For this review, take the finished solid that the model builds, in its own axes (mm). A direction names the side the tool comes from. Round coordinates to 2 decimals unless told otherwise and drop trailing zeros. Write each loop counter-clockwise with the first axis right and the second up, starting at its lowest first coordinate (ties: lowest second). Pieces come first, ordered by that corner, then holes. Notation, with made-up numbers: (32, -16.5) - (78, -16.5) arc R18 ccw to (78, 4.5) - close; hole circle Ø6 at (70, 50.5). An arc over 180 degrees is marked (long way). Answer in a Markdown table with one row per item. Add a question column.
from build123d import *

# Parameters (mm, degrees)
F0_W      = 54.494548589
F0_H      = 39.0236377716
F1_DEPTH  = 5.08
F3_DEPTH  = 12.7
F4_W      = 28.1709115952
F4_H      = 15.8172734082
F4_W_2    = 23.5527232289
F5_DEPTH  = 25.5801105544
F6_W      = 57.7272698283
F6_H      = 25.6309099495
F7_DEPTH  = 25.5801105544
F8_R      = 17.3708251463
F9_DEPTH  = 17.781
F10_DEPTH = 5.08
F12_DEPTH = 7.62


with BuildPart() as f1:
    # F0 (on Top) → F1 (new body)
    with BuildSketch(Plane.XY):
        Rectangle(F0_W, F0_H)
    extrude(amount=F1_DEPTH)

    # F2 (on face) → F3 (join, symmetric)
    with BuildSketch(Plane.XY.offset(5.08)):
        with BuildLine():
            Line((27.2472742945, -19.0345980856), (27.2472742945, 19.0345980856))
            ThreePointArc((27.2472742945, 19.0345980856), (18.7554389024, 0), (27.2472742945, -19.0345980856))
        make_face()
        with BuildLine():
            ThreePointArc((27.2472742945, -19.0345980856), (54.7560079993, -23.3598822472), (69.9136600113, 0))
            ThreePointArc((69.9136600113, 0), (54.7560079993, 23.3598822472), (27.2472742945, 19.0345980856))
            Line((27.2472742945, 19.0345980856), (27.2472742945, -19.0345980856))
        make_face()
    extrude(amount=F3_DEPTH, both=True)

    # F4 (on Front) → F5 (cut, through all)
    with BuildSketch(Plane.XZ):
        with Locations((32.5581813231, -7.9086367041)):
            Rectangle(F4_W, F4_H)
        with Locations((58.4199987352, -7.9086367041)):
            Rectangle(F4_W_2, F4_H)
    extrude(amount=-F5_DEPTH, mode=Mode.SUBTRACT)

    # F6 (on Front) → F7 (cut, through all)
    with BuildSketch(Plane.XZ):
        with Locations((47.5672706962, -12.8154549748)):
            Rectangle(F6_W, F6_H)
    extrude(amount=F7_DEPTH, mode=Mode.SUBTRACT)

    # F8 (on face) → F9 (cut, through all)
    with BuildSketch(Plane.XY.offset(17.78)):
        with Locations((44.3345494568, 0)):
            Circle(F8_R)
    extrude(amount=-F9_DEPTH, mode=Mode.SUBTRACT)

    # F10 (add): a face of the model
    f10_faces = [f1.faces().sort_by_distance(p)[0] for p in [
        (60.9385234936, 18.4962183503, 17.78),
    ]]
    extrude(f10_faces, amount=F10_DEPTH)

    # F11 (on Front) → F12 (join)
    with BuildSketch(Plane.XZ):
        Polygon((18.9776308835, 5.4199039005), (18.9776308835, 22.6603336632), (8.5929688066, 5.4199039005), align=None)
    extrude(amount=F12_DEPTH)


solid = f1.part
Q1. Add section C-C on x = 16.5. State the section outline as (y, z) points, then the cut area to 3 significant figures.
Q2. Insertion check: pin 1 Ø1.3 at (y, z) = (-6, 14.5) entering from +X; pin 2 Ø3 at (x, z) = (56, 4.5) entering from -Y; pin 3 Ø5 at (x, z) = (15.5, 16) entering from -Y. Each pin has a flat end and moves straight along its axis. Give the tip position at first contact, or say it passes through.
Q3. Add section D-D on y = 9. State the section outline as (x, z) points, then the cut area to 3 significant figures.
Q4. Draft analysis for pull direction Z (two halves, no side actions). For faces 1 (the face through (50, -17, 22.86)), 2 (the face through (14, -4, 5.42)), 3 (the face through (-27.247, 0, 3)), state which applies: released by +Z, released by -Z, zero draft, split by the parting line, or undercut.
Q5. Add section A-A on z = 3. State the section outline as (x, y) points.
Q6. Tool access review of faces 4 (the face through (16, 0, 10)), 5 (the face through (0, -19.512, 3)), 6 (the face through (16, -7.62, 10)): name each direction out of +Z, -Z, +X, -X, +Y, -Y from which nothing blocks a thin tool from reaching the whole face with its end or side.
Q7. To check wall thickness, follow probe 1 along X at (y, z) = (0, 4.25); probe 2 along X at (y, z) = (0, 5.25); probe 3 along Z at (x, y) = (5.5, -2). State the ranges of each line that lie inside material, in increasing order.
Q8. Add section B-B on y = -15.5. State the section outline as (x, z) points, then the cut area to 3 significant figures.
Answer sheet:
| question | item | result |
|---|---|---|
| 1 | outline | (-19.51, 0) - (19.51, 0) - (19.51, 5.08) - (-19.51, 5.08) - close; (-7.62, 5.42) - (0, 5.42) - (0, 18.55) - (-7.62, 18.55) - close |
| 1 | area | 298 mm² |
| 2 | pin 1 | stops at x = 69.35 |
| 2 | pin 2 | stops at y = -23.47 |
| 2 | pin 3 | stops at y = -7.62 |
| 3 | outline | (-27.25, 0) - (29.48, 0) - (29.48, 22.86) - (20.39, 22.86) - (20.39, 5.08) - (-27.25, 5.08) - close; (59.19, 0) - (68.28, 0) - (68.28, 22.86) - (59.19, 22.86) - close |
| 3 | area | 657 mm² |
| 4 | face 1 | released by +Z |
| 4 | face 2 | undercut |
| 4 | face 3 | zero draft |
| 5 | outline | (-27.25, -19.51) - (27.25, -19.51) - (27.25, -19.03) arc R25.58 ccw (long way) to (27.25, 19.03) - (27.25, 19.51) - (-27.25, 19.51) - close; hole circle Ø34.74 at (44.33, 0) |
| 6 | face 4 | +Z, -X, +Y |
| 6 | face 5 | +Z, -Z, -X, -Y |
| 6 | face 6 | +Z, -X, -Y |
| 7 | probe 1 | x = -27.25 to 26.96, 61.71 to 69.91 |
| 7 | probe 2 | x = 18.76 to 26.96, 61.71 to 69.91 |
| 7 | probe 3 | z = 0 to 5.08 |
| 8 | outline | (-27.25, 0) - (36.49, 0) - (36.49, 22.86) - (23.99, 22.86) - (23.99, 5.08) - (-27.25, 5.08) - close; (52.18, 0) - (64.68, 0) - (64.68, 22.86) - (52.18, 22.86) - close |
| 8 | area | 832 mm² |
